Design review of the part shown in the three views and the two pictorial views. Dimensions are in mm from the part's minimum x, y and z. A direction names the side the tool comes from. Coordinates: 2 decimals unless noted, no trailing zeros. Write each loop counter-clockwise with the first axis right and the second up, starting at its lowest first coordinate (ties: lowest second). Pieces come first, ordered by that corner, then holes.
Q1. Take a section at D-D, the plane x = 5. Write out the cut boundary in (y, z), plus the area to 3 significant figures.
Q2. Take a section at B-B, the plane x = 8. Write out the cut boundary in (y, z), plus the area to 3 significant figures.
Q3. For L1, parallel to Y at x = 3, z = 5; L2, parallel to Y at x = 4.75, z = 7.5; L3, parallel to Z at x = 9, y = 8.5, list the stretches that pass through material, from the lowest coordinate up.
Q4. For the marked faces 4 and 5, list the 3-axis set-ups (+Z, -Z, +X, -X, +Y, -Y) from which the entire face can be reached by the end or side of a thin tool; tool diameter is ignored.
Q5. Take a section at A-A, the plane z = 5. Write out the cut boundary in (x, y).
Q6. Take a section at C-C, the plane y = 5. Write out the cut boundary in (x, z).
Q7. For pin 1 Ø2 at (x, y) = (5.5, 4.5) entering from -Z; pin 2 Ø4 at (y, z) = (7.5, 7.5) entering from -X; pin 3 Ø3 at (y, z) = (8, 7) entering from +X; pin 4 Ø0.9 at (x, y) = (3, 12.5) entering from -Z, all flat-tipped, find the tip position at first contact; note any pin that passes through.
Q8. The part is to be moulded in two halves that separate along Y. For the marked faces 1, 2 and 3, say which applies: released by +Y, released by -Y, zero draft, split by the parting line, or undercut.
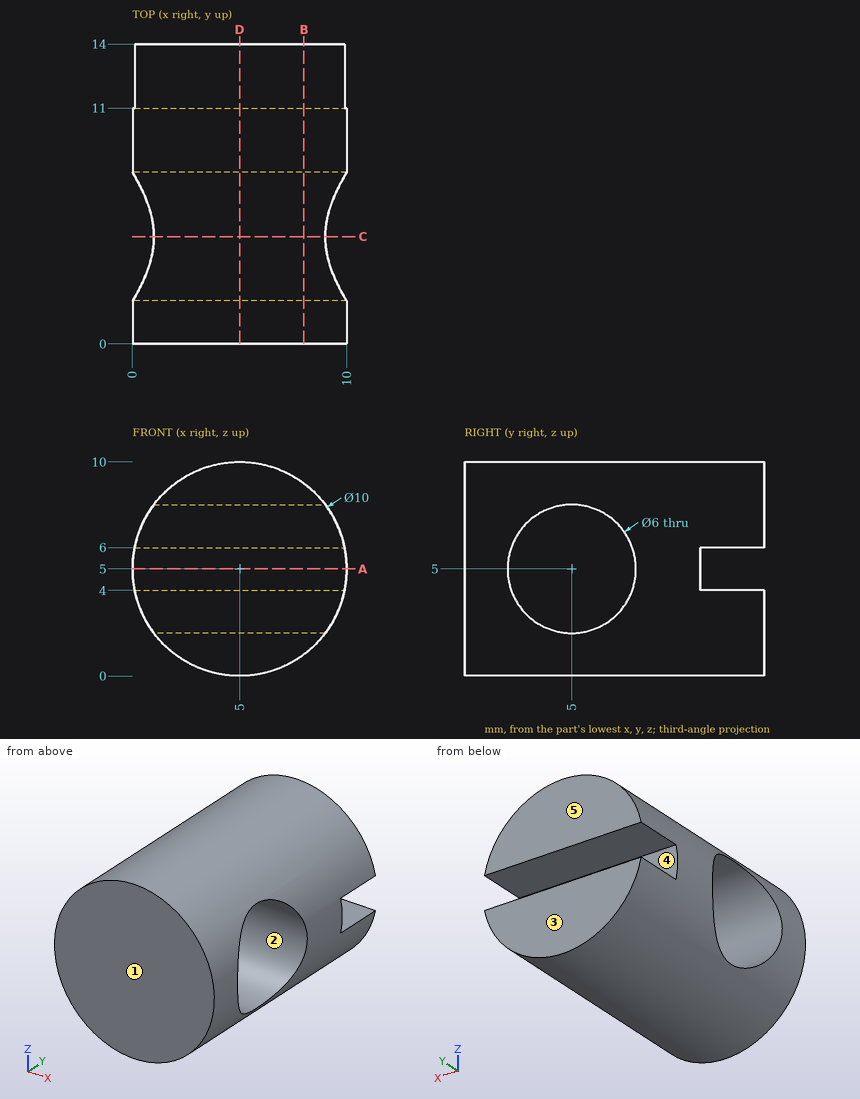
Responses:
1. outline: (0, 0) - (14, 0) - (14, 4) - (11, 4) - (11, 6) - (14, 6) - (14, 10) - (0, 10) - close; hole circle Ø6 at (5, 5)
1. area: 106 mm2
2. outline: (0, 1) - (14, 1) - (14, 4) - (11, 4) - (11, 6) - (14, 6) - (14, 9) - (0, 9) - close; hole circle Ø6 at (5, 5)
2. area: 77.7 mm2
3. L1: y = 0 to 2, 8 to 11
3. L2: y = 0 to 3.34, 6.66 to 14
3. L3: z = 2 to 8
4. face 4: +X, -X, +Y
4. face 5: +Z, -Z, +X, -X, +Y
5. outline: (0, 0) - (10, 0) - (10, 2) - (0, 2) - close; (0, 8) - (10, 8) - (10, 11) - (0, 11) - close
6. outline: (1, 2) arc R5 ccw to (9, 2) - close; (1, 8) - (9, 8) arc R5 ccw to start
7. pin 1: stops at z = 0
7. pin 2: stops at x = 0.03
7. pin 3: stops at x = 9.97
7. pin 4: stops at z = 0.25
8. face 1: released by -Y
8. face 2: undercut
8. face 3: released by +Y
